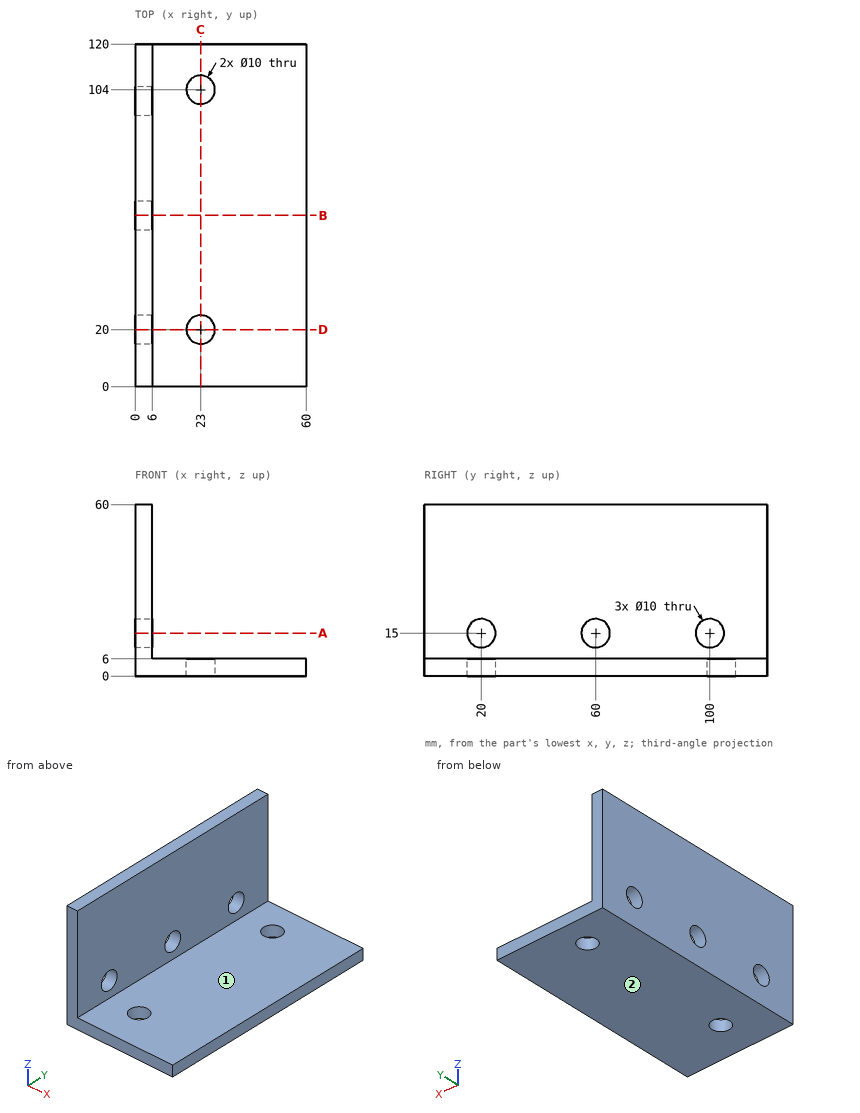
Input: dimensioned drawing with shaded views. Units: mm. Origin: part minimum x, y, z. A direction names the side the tool comes from. Round coordinates to 2 decimals unless told otherwise and drop trailing zeros. Write each loop counter-clockwise with the first axis right and the second up, starting at its lowest first coordinate (ties: lowest second). Pieces come first, ordered by that corner, then holes. Notation, with made-up numbers: (28.5, 83.25) -> (36.5, 83.25) arc R7 cw to (36.5, 87.25) -> close; hole circle Ø1 at (19, 88.25). An arc over 180 degrees is marked (long way). Use CSV: the item, a comma, the result in double quotes. Start each with the question number.
Q1. First-contact query: pin 1 Ø8 at (x, y) = (23, 20) entering from +Z; pin 2 Ø8 at (y, z) = (88.5, 46.5) entering from +X. Flat tips, straight axial feed; report the tip coordinate or a pass-through.
Q2. Section B-B (y = 60). Return loops of the section in (x, z).
Q3. Section C-C (x = 23). Return loops of the section in (y, z), plus the area to 3 significant figures.
Q4. Line query: L1, parallel to Y at x = 23, z = 4.65; L2, parallel to Z at x = 2.75, y = 100; L3, parallel to X at y = 109, z = 40. Output: solid intervals per line, ascending.
Q5. Reachability of the marked faces 1 and 2 from +Z, -Z, +X, -X, +Y, -Y: full face, straight path, thin tool, end or side. Return the list, or none.
Q6. Section D-D (y = 20). Return loops of the section in (x, z).
Q7. Section A-A (z = 15). Return loops of the section in (x, y).
Result sheet:
1,pin 1,"through"
1,pin 2,"x = 6"
2,outline,"(0, 0) -> (60, 0) -> (60, 6) -> (6, 6) -> (6, 10) -> (0, 10) -> close; (0, 20) -> (6, 20) -> (6, 60) -> (0, 60) -> close"
3,outline,"(0, 0) -> (15, 0) -> (15, 6) -> (0, 6) -> close; (25, 0) -> (99, 0) -> (99, 6) -> (25, 6) -> close; (109, 0) -> (120, 0) -> (120, 6) -> (109, 6) -> close"
3,area,"600 mm²"
4,L1,"0 to 15, 25 to 99, 109 to 120"
4,L2,"0 to 10, 20 to 60"
4,L3,"0 to 6"
5,face 1,"+Z, +X, +Y, -Y"
5,face 2,"-Z, +X, -X, +Y, -Y"
6,outline,"(0, 0) -> (18, 0) -> (18, 6) -> (6, 6) -> (6, 10) -> (0, 10) -> close; (0, 20) -> (6, 20) -> (6, 60) -> (0, 60) -> close; (28, 0) -> (60, 0) -> (60, 6) -> (28, 6) -> close"
7,outline,"(0, 0) -> (6, 0) -> (6, 15) -> (0, 15) -> close; (0, 25) -> (6, 25) -> (6, 55) -> (0, 55) -> close; (0, 65) -> (6, 65) -> (6, 95) -> (0, 95) -> close; (0, 105) -> (6, 105) -> (6, 120) -> (0, 120) -> close"
